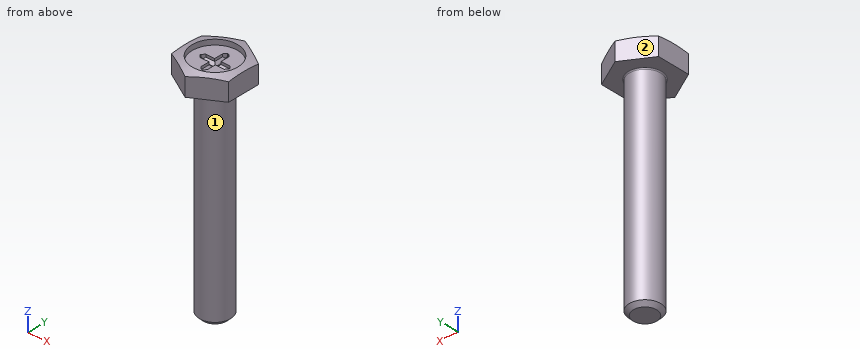
```python
from build123d import *

# Parameters (mm, degrees)
EXTRUDE_1_DEPTH     = 2
SKETCH_3_R          = 1.5
EXTRUDE_3_DEPTH     = 20
SKETCH_7_R          = 2.2
CUT_EXTRUDE_3_DEPTH = 0.5
SKETCH_6_W          = 2.8
SKETCH_6_H          = 0.6
SKETCH_6_W_2        = 0.6
SKETCH_6_H_2        = 2.8
CUT_EXTRUDE_1_DEPTH = 0.5
CHAMFER_1_SIZE      = 0.375
FILLET_1_R          = 0.1
CHAMFER_2_SIZE      = 0.25
CHAMFER_3_SIZE      = 0.25


with BuildPart() as part:
    # 草图1 → 凸台-拉伸1 (new body)
    with BuildSketch(Plane.XY):
        Polygon((0, 3.175426481), (-2.75, 1.58771324), (-2.75, -1.58771324), (0, -3.175426481), (2.75, -1.58771324), (2.75, 1.58771324), align=None)
    extrude(amount=EXTRUDE_1_DEPTH)

    # 草图3 → 凸台-拉伸3 (add)
    with BuildSketch(Plane.XY):
        Circle(SKETCH_3_R)
    extrude(amount=-EXTRUDE_3_DEPTH)

    # 草图4 → 切除-旋转1 (revolve, cut)
    with BuildSketch(Plane(origin=(0, 0, 0), x_dir=(0, 0, -1), z_dir=(1, 0, 0)), mode=Mode.PRIVATE) as cut_revolve_1_sk:
        Polygon((-2, 11), (-2, 2.2), (0.357952893, 11), align=None)
    revolve(cut_revolve_1_sk.sketch.rotate(Axis((0, 0, -2.242017917), (0, 0, 1)), 90), axis=Axis((0, 0, -2.242017917), (0, 0, 1)), mode=Mode.SUBTRACT)

    # 草图7 → 切除-拉伸3 (cut)
    with BuildSketch(Plane.XY.offset(2)):
        Circle(SKETCH_7_R)
    extrude(amount=-CUT_EXTRUDE_3_DEPTH, mode=Mode.SUBTRACT)

    # 草图6 → 切除-拉伸1 (cut)
    with BuildSketch(Plane.XY.offset(1.5)):
        Rectangle(SKETCH_6_W, SKETCH_6_H)
        Rectangle(SKETCH_6_W_2, SKETCH_6_H_2)
    extrude(amount=-CUT_EXTRUDE_1_DEPTH, mode=Mode.SUBTRACT)

    # 倒角1
    chamfer_1_edges = [part.edges().sort_by_distance(p)[0] for p in [
        (-1.5, 0, -20),
    ]]
    chamfer(chamfer_1_edges, length=CHAMFER_1_SIZE)

    # 圆角1
    fillet_1_edges = [part.edges().sort_by_distance(p)[0] for p in [
        (-1.5, 0, 0),
    ]]
    fillet(fillet_1_edges, radius=FILLET_1_R)

    # 倒角2
    chamfer_2_edges = [part.edges().sort_by_distance(p)[0] for p in [
        (0.3, 0.85, 1),
        (0.85, 0.3, 1),
        (-0.3, -0.85, 1),
        (-1.4, 0, 1),
        (-0.85, 0.3, 1),
        (-0.3, 0.85, 1),
        (0, 1.4, 1),
        (0, -1.4, 1),
        (0.3, -0.85, 1),
        (-0.85, -0.3, 1),
        (1.4, 0, 1),
        (0.85, -0.3, 1),
    ]]
    chamfer(chamfer_2_edges, length=CHAMFER_2_SIZE)

    # 倒角3
    chamfer_3_edges = [part.edges().sort_by_distance(p)[0] for p in [
        (1.4, 0.3, 1.375),
        (1.4, -0.3, 1.375),
        (0.3, -1.4, 1.375),
        (-0.3, -1.4, 1.375),
        (-1.4, -0.3, 1.375),
        (-1.4, 0.3, 1.375),
        (-0.3, 1.4, 1.375),
        (0.3, 1.4, 1.375),
    ]]
    chamfer(chamfer_3_edges, length=CHAMFER_3_SIZE)


solid = part.part
```
CAD build for the part. Positions are in the model's coordinates, mm. Face numbers are marked on the shaded views. A direction names the side the tool comes from. Coordinates: 2 decimals unless noted, no trailing zeros. Order: outer loops, then holes, each group sorted by start corner. A loop starts at its lowest first (then second) coordinate and runs counter-clockwise, first axis right, second up. Notation, with made-up numbers: M -28.5,-23.75 L 16.5,-23.75 A22 ccw 16.5,-8.75 Z; hole C 55,-23.75 d10. An arc over 180 degrees is marked long. Write each question's results on one line, items separated by ' | '. Start each with the question number.
Q1. Cut at A-A (z = -8.25). List the corners of the cut face in (x, y).
Q2. Which spindle directions (+Z, -Z, +X, -X, +Y, -Y) get a long thin tool onto all of the face, cutting with end or side? Do the marked faces 1 and 2. Say none if no direction does.
Q3. Drill centre lines: probe 1 along Y at (x, z) = (0, -7.5); probe 2 along Z at (x, y) = (-0.55, 2); probe 3 along Z at (x, y) = (-0.35, -1). Where is each one in solid material? Low to high. Write a range as from..to.
Q4. Flat gauge pins, fed straight in: P1, Ø1.5, axis at x = -1.5, y = 0.5, coming from the +Z side; P2, Ø2, axis at y = -2, z = -16, coming from the +X side; P3, Ø0.7, axis at x = 0.5, y = 0.5, coming from the +Z side; P4, Ø1.5, axis at x = 1.5, z = -8, coming from the +Y side. Where does each tip first touch, or does it go through?
Found:
1) outline: C 0,0 d3
2) face 1: -Z | face 2: +Z, -Z, -X, +Y
3) probe 1: -1.5..1.5 | probe 2: 0..1.5 | probe 3: -20..1.5
4) P1: z = 2 | P2: x = 1.12 | P3: z = 1.5 | P4: y = 1.3
